from build123d import *

# Parameters (mm, degrees)
F0_W     = 10
F0_H     = 16
F1_DEPTH = 2
F2_W     = 1.5
F2_H     = 6
F2_W_2   = 6
F2_H_2   = 1.5
F3_DEPTH = 2
F4_SIZE  = 0.7


with BuildPart() as f1:
    # F0 (on Top) → F1 (new body)
    with BuildSketch(Plane.XY):
        Rectangle(F0_W, F0_H)
    extrude(amount=-F1_DEPTH)

    # F2 (on face) → F3 (join)
    with BuildSketch(Plane.XY):
        with Locations((-3.987426, 3.969108)):
            Rectangle(F2_W, F2_H)
        with Locations((0, 6.868761)):
            Rectangle(F2_W_2, F2_H_2)
        with Locations((3.987426, 3.969108)):
            Rectangle(F2_W, F2_H)
        with Locations((0.028471, 0.005555)):
            Rectangle(F2_W_2, F2_H_2)
        with Locations((-3.987426, -3.969108)):
            Rectangle(F2_W, F2_H)
        with Locations((0, -6.868761)):
            Rectangle(F2_W_2, F2_H_2)
        with Locations((3.987426, -3.969108)):
            Rectangle(F2_W, F2_H)
    extrude(amount=F3_DEPTH)

    # F4
    f4_edges = [f1.edges().sort_by_distance(p)[0] for p in [
        (3, 6.118761, 1),
        (3.237426, 6.969108, 1),
        (3.237426, 0.969108, 1),
        (4.737426, 0.969108, 1),
        (3.237426, -0.969108, 1),
        (3.028471, -0.744445, 1),
        (-2.971529, -0.744445, 1),
        (-2.971529, 0.755555, 1),
        (-3.237426, 0.969108, 1),
        (-4.737426, 0.969108, 1),
        (-4.737426, 6.969108, 1),
        (-3, 6.118761, 1),
        (-3, 7.618761, 1),
        (3.237426, -6.969108, 1),
        (4.737426, -6.969108, 1),
        (3, -7.618761, 1),
        (-3, -7.618761, 1),
        (-3.237426, -6.969108, 1),
        (-4.737426, -6.969108, 1),
        (-3, -6.118761, 1),
        (-4.737426, -0.969108, 1),
        (-3.237426, -0.969108, 1),
        (3.028471, 0.755555, 1),
        (4.737426, -0.969108, 1),
        (3, -6.118761, 1),
        (4.737426, 6.969108, 1),
        (3, 7.618761, 1),
        (-3.237426, 6.969108, 1),
    ]]
    chamfer(f4_edges, length=F4_SIZE)


solid = f1.part
Part model, mm, in its own coordinate system. A direction names the side the tool comes from. Coordinates: 2 decimals unless noted, no trailing zeros. Order: outer loops, then holes, each group sorted by start corner. A loop starts at its lowest first (then second) coordinate and runs counter-clockwise, first axis right, second up.
(1) Pull direction Y, two halves, no side cores. Call faces 1 (the face through (0, 6.119, 1)), 2 (the face through (-4.737, -4, 1)), 3 (the face through (0, -7.619, 1)): pulls with the +Y half, pulls with the -Y half, needs draft (parallel to the pull), parting line crosses it, or undercut.
Check sheet entries:
face 1: undercut
face 2: needs draft
face 3: pulls with the -Y half
(2) Slice it at C-C, the plane z = 1.5. State how many separate pieces and enclosed holes the cut face has, and give its area (3 significant figures).
Check sheet entries:
separate pieces: 7
enclosed holes: 0
area: 56.1 mm2
(3) Slice it at D-D, the plane x = 4.25. Write the cut outline in (y, z).
Check sheet entries:
outline: (-8, -2) - (8, -2) - (8, 0) - (6.76, 0) - (6.76, 2) - (1.18, 2) - (1.18, 0) - (-1.18, 0) - (-1.18, 2) - (-6.76, 2) - (-6.76, 0) - (-8, 0) - close
(4) Probe L1, parallel to Y at x = 0.75, z = 1; L2, parallel to X at y = -2.25, z = 0.45; L3, parallel to X at y = 6.75, z = 1.8. List the from-to ranges inside material, lowest first.
Check sheet entries:
L1: y = -7.62 to -6.12, -0.74 to 0.76, 6.12 to 7.62
L2: x = -4.74 to -3.24, 3.24 to 4.74
L3: x = -4.26 to -3.72, -2.93 to 2.93, 3.72 to 4.26
(5) Pin check, flat tips, straight feed: pin 1 Ø2 at (y, z) = (-4, 1.5) entering from +X; pin 2 Ø0.6 at (x, z) = (1, 0.5) entering from +Y; pin 3 Ø0.6 at (x, z) = (1, 1) entering from -Y. Stop position of each tip, or through.
Check sheet entries:
pin 1: stops at x = 4.74
pin 2: stops at y = 7.62
pin 3: stops at y = -7.62
(6) Slice it at B-B, the plane x = -2. Write the cut outline in (y, z).
Check sheet entries:
outline: (-8, -2) - (8, -2) - (8, 0) - (7.62, 0) - (7.62, 2) - (6.12, 2) - (6.12, 0) - (0.76, 0) - (0.76, 2) - (-0.74, 2) - (-0.74, 0) - (-6.12, 0) - (-6.12, 2) - (-7.62, 2) - (-7.62, 0) - (-8, 0) - close
(7) Slice it at A-A, the plane y = -2.5. Write the cut outline in (x, z).
Check sheet entries:
outline: (-5, -2) - (5, -2) - (5, 0) - (4.74, 0) - (4.74, 2) - (3.24, 2) - (3.24, 0) - (-3.24, 0) - (-3.24, 2) - (-4.74, 2) - (-4.74, 0) - (-5, 0) - close
(8) Tool access for faces 4 (the face through (0, 2, 0)), 5 (the face through (0, -0.744, 1)), 6 (the face through (4.737, -4, 1)), 7 (the face through (-3.237, 4, 1)): list every direction of +Z, -Z, +X, -X, +Y, -Y with a clear straight run to the whole face (end or side of a thin tool).
Check sheet entries:
face 4: +Z
face 5: +Z, +X, -X
face 6: +Z, +X, +Y, -Y
face 7: +Z, +Y, -Y
